Here's how the part is built. I have some questions about the finished solid (model axes, mm). Face numbers are marked on the shaded views. A direction names the side the tool comes from. Give positions to 0.01 mm unless a question says otherwise; leave off trailing zeros. Loops run counter-clockwise (first coordinate to the right, second up) from the corner with the lowest first, then second, coordinate; pieces in that order, holes last. Notation, with made-up numbers: M -38,25 L -18,25 A31 cw -18,56 Z; hole C 40,20.25 d9. An arc over 180 degrees is marked long. Write item = value, one per line. Start each with the question number.
```python
from build123d import *

# Parameters (mm, degrees)
F1_DEPTH = 63.5
F2_DEPTH = 25.4


with BuildPart() as f1:
    # F0 (on Front) → F1 (new body, symmetric)
    with BuildSketch(Plane.XZ):
        Polygon((-41.275, -9.525), (41.275, -9.525), (41.275, -7.805796), (41.275, 9.525), (22.225, 9.525), (-41.275, 9.525), align=None)
    extrude(amount=F1_DEPTH, both=True)

    # F0 (on Front) → F2 (join)
    with BuildSketch(Plane.XZ):
        Polygon((-41.275, -9.525), (41.275, -9.525), (41.275, -7.805796), (41.275, 9.525), (22.225, 9.525), (-41.275, 9.525), align=None)
        with BuildLine():
            add(Edge.make_bspline(
                [(-41.275, 9.525), (-41.482281, 52.308347), (19.065714, 62.464789), (51.622058, 61.9252)],
                knots=[0, 0, 0, 0, 106.656666, 106.656666, 106.656666, 106.656666], degree=3))
            Line((-41.275, 9.525), (22.225, 9.525))
            Line((22.225, 9.525), (22.225, 32.528142))
            ThreePointArc((22.225, 32.528142), (30.835199, 53.315001), (51.622058, 61.9252))
        make_face()
        with BuildLine():
            Line((22.225, 9.525), (41.275, 9.525))
            Line((41.275, 9.525), (41.275, 32.528142))
            ThreePointArc((41.275, 32.528142), (44.305583, 39.844617), (51.622058, 42.8752))
            Line((51.622058, 42.8752), (60.325, 42.8752))
            Line((60.325, 42.8752), (60.325, 61.9252))
            Line((60.325, 61.9252), (51.622058, 61.9252))
            ThreePointArc((51.622058, 61.9252), (30.835199, 53.315001), (22.225, 32.528142))
            Line((22.225, 32.528142), (22.225, 9.525))
        make_face()
        Polygon((60.325, 66.675), (60.325, 61.9252), (60.325, 42.8752), (60.325, 38.1), (82.32934, 38.1), (82.312385, 66.675), align=None)
        Polygon((111.125, 66.675), (82.312385, 66.675), (82.32934, 38.1), (111.125, 38.1), align=None)
    extrude(amount=F2_DEPTH)


solid = f1.part
```
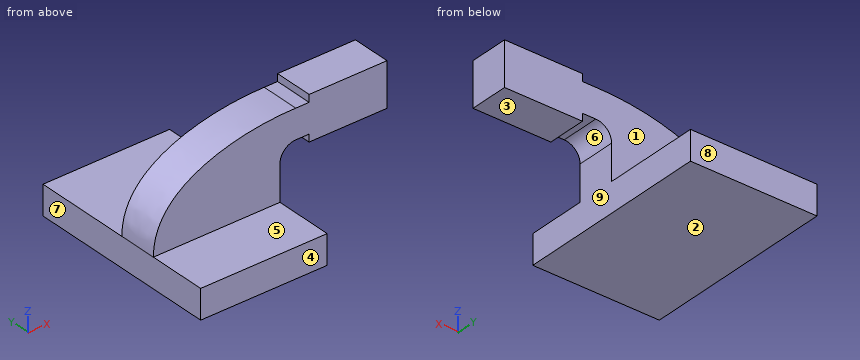
Q1. We'd pull the mould along X, two halves only. Please class the marked faces 6, 7, 8 and 9: pulls with the +X half, pulls with the -X half, needs draft (parallel to the pull), parting line crosses it, or undercut.
Q2. On a 3-axis mill with a long thin cutter (end or side, diameter ignored), from which of +Z, -Z, +X, -X, +Y, -Y can I reach the whole of each face in a straight line? I mean the marked faces 1, 2, 3, 4 and 5. Say none if no direction works.
Q3. If we section it at B-B, the plane y = 7: List the corners of the cut face in (x, z) for me (3 decimals).
Q4. If we section it at A-A, the plane z = 2: List the corners of the cut face in (x, y) for me (3 decimals), then the cut area to 3 significant figures.
Q5. If I drill on line 1 along X through (y, z) = (2, 2) (3 decimals); line 2 along Y through (x, z) = (80, 58); line 3 along Z through (x, y) = (-28, -54) (3 decimals), over which ranges is the centre line in solid material (lowest first)?
Q6. Will these pins go through, and if not, where does the flat tip stop? pin 1 (5.5 mm diameter, centred on y = -12.5, z = 41.5, fed in from -X); pin 2 (5 mm diameter, centred on x = -10.5, y = -29, fed in from +Z) (3 decimals); pin 3 (7 mm diameter, centred on x = 56.5, y = -10.5, fed in from +Z).
Resolved:
q1.face_6 = undercut
q1.face_7 = pulls with the -X half
q1.face_8 = needs draft
q1.face_9 = pulls with the +X half
q2.face_1 = +Z, +X, -X, +Y
q2.face_2 = -Z, +X, -X, +Y, -Y
q2.face_3 = -Z, +X, +Y, -Y
q2.face_4 = +Z, -Z, +X, -X, -Y
q2.face_5 = +Z, +X, -X, -Y
q3.outline = M -41.275,-9.525 L 41.275,-9.525 L 41.275,9.525 L -41.275,9.525 Z
q4.outline = M -41.275,-63.5 L 41.275,-63.5 L 41.275,63.5 L -41.275,63.5 Z
q4.area = 10,500 mm²
q5.line_1 = -41.275 to 41.275
q5.line_2 = -25.4 to 0
q5.line_3 = -9.525 to 9.525
q6.pin_1 = -28.61
q6.pin_2 = 9.525
q6.pin_3 = 61.93
